Autodesk Fusion 360 part; units mm, degrees
sketch "Sketch 1" plane through (0, 0, 0) normal (0, 1, 0) x (-1, 0, 0)
  line L0 (0.207, 14.4246) -> (-14.793, 14.4246)
  line L1 (0.207, 64.4246) -> (0.207, 14.4246)
  line L2 (-14.793, 14.4246) -> (-14.793, 64.4246)
  line L3 (-14.793, 64.4246) -> (0.207, 64.4246)
  line L4 (-92.925, 5.6402) -> (-78.1529, 8.2449)
  line L5 (-78.1529, 8.2449) -> (-89.7874, 74.227)
  line L6 (-104.5595, 71.6223) -> (-92.925, 5.6402)
  line L7 (-89.7874, 74.227) -> (-104.5595, 71.6223)
  circle A0 centre (-94.793, 59.4246) radius 4
  circle A1 centre (-87.7399, 19.4246) radius 4
  line L8 (0.207, 4.4246) -> (-114.793, 4.4246)
  line L9 (-114.793, 4.4246) -> (-114.793, 74.4246)
  line L10 (-114.793, 74.4246) -> (0.207, 74.4246)
  line L11 (0.207, 74.4246) -> (0.207, 4.4246)
  line L12 (0.207, 74.4246) -> (10, 74.4246)
  line L13 (10, 74.4246) -> (10, 44.4246)
  line L14 (10, 44.4246) -> (0.207, 44.4246)
  line L15 (0.207, 44.4246) -> (0.207, 74.4246)
  line L16 (-24.793, 67.4246) -> (-104.793, 67.4246)
  line L17 (-104.793, 67.4246) -> (-104.793, 51.4246)
  line L18 (-104.793, 51.4246) -> (-24.793, 51.4246)
  line L19 (-24.793, 51.4246) -> (-24.793, 67.4246)
  line L20 (-24.793, 27.4246) -> (-104.793, 27.4246)
  line L21 (-104.793, 27.4246) -> (-104.793, 11.4246)
  line L22 (-104.793, 11.4246) -> (-24.793, 11.4246)
  line L23 (-24.793, 11.4246) -> (-24.793, 27.4246)
  line L24 (-24.793, 51.4246) -> (-104.793, 51.4246)
  line L25 (-104.793, 51.4246) -> (-104.793, 59.4246)
  line L26 (-104.793, 59.4246) -> (-24.793, 59.4246)
  line L27 (-24.793, 59.4246) -> (-24.793, 51.4246)
  line L28 (-24.793, 11.4246) -> (-104.793, 11.4246)
  line L29 (-104.793, 11.4246) -> (-104.793, 19.4246)
  line L30 (-104.793, 19.4246) -> (-24.793, 19.4246)
  line L31 (-24.793, 19.4246) -> (-24.793, 11.4246)
  circle A2 centre (-30.793, 59.4246) radius 4
  circle A3 centre (-40.3644, 59.4246) radius 4
  circle A4 centre (-49.9359, 59.4246) radius 4
  circle A5 centre (-59.5073, 59.4246) radius 4
  circle A6 centre (-69.0787, 59.4246) radius 4
  circle A7 centre (-78.6501, 59.4246) radius 4
  circle A8 centre (-88.2216, 59.4246) radius 4
  circle A9 centre (-97.793, 59.4246) radius 4
  circle A10 centre (-30.793, 19.4246) radius 4
  circle A11 centre (-40.3644, 19.4246) radius 4
  circle A12 centre (-49.9359, 19.4246) radius 4
  circle A13 centre (-59.5073, 19.4246) radius 4
  circle A14 centre (-69.0787, 19.4246) radius 4
  circle A15 centre (-78.6501, 19.4246) radius 4
  circle A16 centre (-88.2216, 19.4246) radius 4
  circle A17 centre (-97.793, 19.4246) radius 4
  point P0 (-97.1734, 72.9246)
  dimension "d9" = 15
  dimension "d10" = 50
  dimension "d11" = 15
  dimension "d12" = 67
  dimension "d13" = 8
  dimension "d14" = 7.5
  dimension "d15" = 8
  dimension "d17" = 7.5
  dimension "d18" = 40
  dimension "d19" = 13.5
  dimension "d22" = 10
  dimension "d23" = 10
  dimension "d24" = 80
  dimension "d25" = 100
  dimension "d27" = 30
  dimension "d28" = 80
  dimension "d29" = 16
  dimension "d30" = 10
  dimension "d31" = 80
  dimension "d32" = 16
  dimension "d33" = 10
  dimension "d35" = 10
  dimension "d36" = 8
  dimension "d37" = 8
  dimension "d38" = 7
  dimension "d39" = 8
  dimension "d42" = -67
  dimension "d43" = 0
  dimension "d44" = 6
  dimension "d45" = 8
  dimension "d46" = 6
  dimension "d49" = -67
  dimension "d50" = 0
extrude "Extrude3" add sketch "Sketch 1" along normal blind 200 contours L0 L1 L2 L3 L11 L15 | L4 L5 L6 L22 L28 | L5 L6 A1 L22 L28 L30 A15 A16 A17 | L6 L30 A17 | L5 L30 A15 | L6 L30 A17 | L5 L6 A1 L20 L30 A15 A16 A17 | L5 L30 A15 | A1 L30 A16 | A1 L30 A16 | L5 L6 L18 L20 L24 | L5 L6 A0 L18 L24 L26 A8 A9 | L5 L6 A0 L16 L26 A8 A9 | L5 A0 L26 A8 | L5 L6 L7 L16 | A0 L26 A9 | A0 L26 A9 | L5 A0 L26 A8 picked at (-94.3244, 19.2578) picked at (-81.7956, 19.242) picked at (-94.3265, 19.6077) picked at (-81.7939, 19.6192) picked at (-91.9756, 20.1938) picked at (-91.9756, 18.6555) picked at (-99.7654, 59.8073) picked at (-99.7654, 59.042) makes body 1 at (14.793, 66.6667, 31.0913) makes body 2 at (100.6813, 66.6667, 49.6282)
extrude "Extrude4" add sketch "Sketch 1" along normal blind 10 separate body contours L0 L2 L3 L8 L9 L10 L11 L15 | L1 L11 L12 L13 L14 L15 | L4 L5 L6 L22 L28 | L6 L21 L22 L28 L29 L30 A17 | L5 L6 A1 L22 L28 L30 A15 A16 A17 | L5 L22 L23 L28 L30 L31 A10 A11 A12 A13 A14 A15 | L6 L30 A17 | L6 L30 A17 | L5 L30 A15 | L5 L30 A15 | L6 L30 A17 | L6 L30 A17 | L6 L20 L21 L30 A17 | L5 L6 A1 L20 L30 A15 A16 A17 | L5 L30 A15 | L5 L30 A15 | L5 L20 L23 L30 A10 A11 A12 A13 A14 A15 | A1 L30 A16 | A1 L30 A16 | A1 L30 A16 | A1 L30 A16 | L30 A14 | L30 A14 | L30 A10 | L30 A10 | L5 L6 L18 L20 L24 | A1 L30 A16 | A1 L30 A16 | L6 L17 L18 L24 L25 L26 | L5 L6 A0 L18 L24 L26 A8 A9 | L5 L18 L19 L24 L26 L27 A2 A3 A4 A5 A6 A7 A8 | L30 A13 | L30 A13 | L30 A11 | L30 A11 | L6 L16 L17 L26 | L5 L6 A0 L16 L26 A8 A9 | L5 A0 L26 A8 | L5 L26 A8 | L5 L6 L7 L16 | A0 L26 A9 | A0 L26 A9 | L5 A0 L26 A8 | L5 L26 A8 | A0 L26 A8 | A0 L26 A8 A9 | L5 L16 L19 L26 A2 A3 A4 A5 A6 A7 A8 | L30 A12 | L30 A12 | A0 L26 A9 | A0 L26 A9 | A0 L26 A8 A9 | A0 L26 A8 | L26 A7 | L26 A7 | L26 A2 | L26 A2 | L26 A6 | L26 A6 | L26 A3 | L26 A3 | L26 A5 | L26 A5 | L26 A4 | L26 A4 makes body 3
extrude "Extrude5" cut sketch "Sketch 1" along normal blind 4 from surface at 6 contours L6 L16 L17 L26 | L5 L6 A0 L16 L26 A8 A9 | L5 A0 L26 A8 | L5 L26 A8 | A0 L26 A9 | A0 L26 A9 | L5 A0 L26 A8 | L5 L26 A8 | A0 L26 A8 | L5 L16 L19 L26 A2 A3 A4 A5 A6 A7 A8 | A0 L26 A9 | A0 L26 A9 | A0 L26 A8 A9 | A0 L26 A8 | L26 A7 | L26 A7 | L26 A2 | L26 A2 | L26 A6 | L26 A6 | L26 A3 | L26 A3 | L26 A5 | L26 A5 | L26 A4 | L26 A4 picked at (-92.8229, 61.5231) bodies 3
extrude "Extrude6" cut sketch "Sketch 1" along normal blind 4 from surface at 6 contours L6 L30 A17 | L6 L30 A17 | L5 L30 A15 | L5 L30 A15 | L6 L30 A17 | L6 L30 A17 | L6 L20 L21 L30 A17 | L5 L6 A1 L20 L30 A15 A16 A17 | L5 L30 A15 | L5 L30 A15 | L5 L20 L23 L30 A10 A11 A12 A13 A14 A15 | A1 L30 A16 | A1 L30 A16 | A1 L30 A16 | L30 A14 | L30 A14 | L30 A10 | L30 A10 | A1 L30 A16 | A1 L30 A16 | L30 A13 | L30 A13 | L30 A11 | L30 A11 | L30 A12 | L30 A12 picked at (-91.9756, 20.1938) picked at (-91.9756, 18.6555) picked at (-83.9859, 20.1938) picked at (-89.2213, 19.2421) picked at (-89.2213, 19.6072) bodies 3
hidden bodies 1 2
Source: CAD feature listing. Evaluate the final solid. Frame: model axes, mm. A direction names the side the tool comes from. Round coordinates to 2 decimals unless told otherwise and drop trailing zeros. Loops run counter-clockwise (first coordinate to the right, second up) from the corner with the lowest first, then second, coordinate; pieces in that order, holes last.
Q1. Ray query, line 1 (X direction, y = 4.5, z = 58); line 2 (Z direction, x = 53, y = 9.5); line 3 (Z direction, x = 100, y = 9). Return the intervals inside material, ascending.
Q2. Section D-D, the plane y = 8.5. State how many separate pieces and enclosed holes the cut face has, plus the area to 3 significant figures.
Q3. Section B-B, the plane z = 23. Return loops of the section in (x, y), plus the area to 3 significant figures.
Q4. Access query for faces 4 (the face through (56, 5, 4.425)), 5 (the face through (7, 5, 14.425)), 6 (the face through (-5, 5, 44.425)), 7 (the face through (40.276, 7.972, 15.426)). Directions: +Z, -Z, +X, -X, +Y, -Y. A direction counts if a zero-diameter tool reaches every point of the face in a straight line with its end or side. Return the directions, or none.
Q5. Section A-A, the plane y = 2.5. Return loops of the section in (x, z).
Q6. Section C-C, the plane x = 68. Return loops of the section in (y, z), plus the area to 3 significant figures.
Q7. Mould query, pull axis X, two halves, no side actions, for faces 1 (the face through (-10, 5, 60)), 2 (the face through (53, 5, 74.425)), 3 (the face through (97.705, 7.972, 15.426)). Classes: pulls with the +X half, pulls with the -X half, needs draft (parallel to the pull), parting line crosses it, or undercut.
Solutions:
1. line 1: x = -10 to -0.21, 14.79 to 114.79
1. line 2: z = 4.42 to 16.85, 27.42 to 56.85, 67.42 to 74.42
1. line 3: z = 4.42 to 16.09, 27.42 to 56.09, 67.42 to 74.42
2. separate pieces: 1
2. enclosed holes: 2
2. area: 5,910 mm2
3. outline: (14.79, 0) - (114.79, 0) - (114.79, 10) - (104.79, 10) - (104.79, 6) - (24.79, 6) - (24.79, 10) - (14.79, 10) - close
3. area: 680 mm2
4. face 4: -Z, +X, -X, +Y, -Y
4. face 5: -X, +Y, -Y
4. face 6: -Z, -X, +Y, -Y
4. face 7: +Y
5. outline: (-10, 44.42) - (-0.21, 44.42) - (-0.21, 64.42) - (14.79, 64.42) - (14.79, 14.42) - (-0.21, 14.42) - (-0.21, 4.42) - (114.79, 4.42) - (114.79, 74.42) - (-10, 74.42) - close
6. outline: (0, 4.42) - (10, 4.42) - (10, 15.57) - (6, 15.57) - (6, 27.42) - (10, 27.42) - (10, 55.57) - (6, 55.57) - (6, 67.42) - (10, 67.42) - (10, 74.42) - (0, 74.42) - close
6. area: 605 mm2
7. face 1: pulls with the -X half
7. face 2: needs draft
7. face 3: undercut
